```python
from build123d import *

# Parameters (mm, degrees)
BOSS_EXTRUDE1_DEPTH = 4.9784
SKETCH3_R           = 4.3434
SKETCH3_R_2         = 2.794
BOSS_EXTRUDE2_DEPTH = 2.921
CUT_EXTRUDE1_REACH  = 5.264
SKETCH4_R           = 1.397


with BuildPart() as part:
    # Sketch2 → Boss-Extrude1 (new body, symmetric)
    with BuildSketch(Plane.XY):
        Polygon((-3.8227, 0), (-4.9911, 0), (-4.9911, 3.2639), (4.9911, 3.2639), (4.9911, 0), (3.8227, 0), (3.8227, 2.0955), (-3.8227, 2.0955), align=None)
    extrude(amount=BOSS_EXTRUDE1_DEPTH, both=True)

    # Sketch3 → Boss-Extrude2 (add)
    with BuildSketch(Plane(origin=(0, 3.2639, 0), x_dir=(1, 0, 0), z_dir=(0, 1, 0))):
        Circle(SKETCH3_R)
        Circle(SKETCH3_R_2, mode=Mode.SUBTRACT)
    extrude(amount=BOSS_EXTRUDE2_DEPTH)

    # Sketch4 → Cut-Extrude1 (cut, up to next)
    with BuildSketch(Plane(origin=(0, 3.2639, 0), x_dir=(1, 0, 0), z_dir=(0, 1, 0)), mode=Mode.PRIVATE) as cut_extrude1_sk1:
        Circle(SKETCH4_R)
    cut_extrude1_tool1 = extrude(cut_extrude1_sk1.sketch, amount=-CUT_EXTRUDE1_REACH, mode=Mode.PRIVATE) & part.part
    add(cut_extrude1_tool1.solids().sort_by_distance((0, 3.2639, 0))[0], mode=Mode.SUBTRACT)


solid = part.part
```
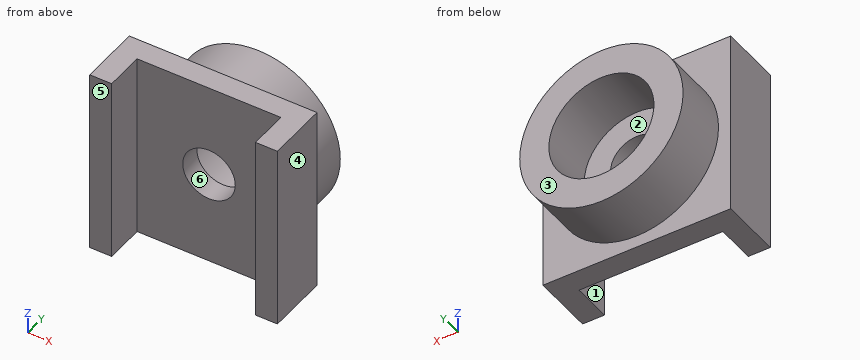
Work out the finished part from the listing and answer in its coordinate system (mm). Face numbers are marked on the shaded views. A direction names the side the tool comes from. Give positions to 0.01 mm unless a question says otherwise; leave off trailing zeros. Order: outer loops, then holes, each group sorted by start corner. A loop starts at its lowest first (then second) coordinate and runs counter-clockwise, first axis right, second up. Notation, with made-up numbers: (11.5, -20.75) -> (21.5, -20.75) arc R15 cw to (21.5, 7.25) -> close; hole circle Ø8 at (18.25, 76). An arc over 180 degrees is marked (long way). Answer as CSV lines item,"result". Start each with the question number.
(1) For a pull along X with two mould halves and no side action, classify the marked faces 4, 5 and 6 as released by +X, released by -X, zero draft, split by the parting line, or undercut.
(2) Section D-D, the plane y = 3 is taken. Write down the section's boundary in (x, z).
(3) Section C-C, the plane x = 0 is taken. Write down the section's boundary in (y, z), plus the area to 3 significant figures.
(4) Each of these flat-tipped pins is pushed along its axis until it touches: pin 1 Ø4.5 at (x, z) = (0, 0) entering from +Y; pin 2 Ø1 at (x, z) = (-2.5, 0) entering from +Y; pin 3 Ø2 at (y, z) = (4.5, -3.5) entering from +X; pin 4 Ø4 at (x, z) = (-1, 0.5) entering from -Y. Where does it stop, or does it pass through?
(5) Which of the six approach directions +Z, -Z, +X, -X, +Y, -Y give full straight-line access (tool end or side, diameter ignored) to the marked faces 1, 2 and 3?
(6) Section B-B, the plane y = 1.75 is taken. Write down the section's boundary in (x, z), plus the area to 3 significant figures.
(7) Consider line 1 along X through (y, z) = (1.5, -2.75); line 2 along Z through (x, y) = (0, 2.7); line 3 along X through (y, z) = (5.5, 0). Determine where each line is inside the solid, lowest interval first.
(8) Section A-A, the plane z = 0 is taken. Write down the section's boundary in (x, y), plus the area to 3 significant figures.
Entries:
1,face 4,"released by +X"
1,face 5,"zero draft"
1,face 6,"undercut"
2,outline,"(-4.99, -4.98) -> (4.99, -4.98) -> (4.99, 4.98) -> (-4.99, 4.98) -> close; hole circle Ø2.79 at (0, 0)"
3,outline,"(2.1, -4.98) -> (3.26, -4.98) -> (3.26, -4.34) -> (6.18, -4.34) -> (6.18, -2.79) -> (3.26, -2.79) -> (3.26, -1.4) -> (2.1, -1.4) -> close; (2.1, 1.4) -> (3.26, 1.4) -> (3.26, 2.79) -> (6.18, 2.79) -> (6.18, 4.34) -> (3.26, 4.34) -> (3.26, 4.98) -> (2.1, 4.98) -> close"
3,area,"17.4 mm²"
4,pin 1,"y = 3.26"
4,pin 2,"y = 6.18"
4,pin 3,"x = 3.55"
4,pin 4,"y = 2.1"
5,face 1,"+Z, -Z, -Y"
5,face 2,"+Y"
5,face 3,"+Z, -Z, +X, -X, +Y"
6,outline,"(-4.99, -4.98) -> (-3.82, -4.98) -> (-3.82, 4.98) -> (-4.99, 4.98) -> close; (3.82, -4.98) -> (4.99, -4.98) -> (4.99, 4.98) -> (3.82, 4.98) -> close"
6,area,"23.3 mm²"
7,line 1,"-4.99 to -3.82, 3.82 to 4.99"
7,line 2,"-4.98 to -1.4, 1.4 to 4.98"
7,line 3,"-4.34 to -2.79, 2.79 to 4.34"
8,outline,"(-4.99, 0) -> (-3.82, 0) -> (-3.82, 2.1) -> (-1.4, 2.1) -> (-1.4, 3.26) -> (-2.79, 3.26) -> (-2.79, 6.18) -> (-4.34, 6.18) -> (-4.34, 3.26) -> (-4.99, 3.26) -> close; (1.4, 2.1) -> (3.82, 2.1) -> (3.82, 0) -> (4.99, 0) -> (4.99, 3.26) -> (4.34, 3.26) -> (4.34, 6.18) -> (2.79, 6.18) -> (2.79, 3.26) -> (1.4, 3.26) -> close"
8,area,"22.3 mm²"
